Autodesk Inventor part; units mm, degrees
ref_plane "YZ Plane" through (0, 0, 0) normal (1, 0, 0) x (0, 1, 0)
ref_plane "XZ Plane" through (0, 0, 0) normal (0, 1, 0) x (-1, 0, 0)
ref_plane "XY Plane" through (0, 0, 0) normal (0, 0, 1) x (1, 0, 0)
sketch "Sketch1" plane through (0, 0, 0) normal (0, 0, 1) x (1, 0, 0)
  line L0 (0, 0) -> (152.4, 0)
  line L1 (152.4, 0) -> (152.4, 3.175)
  line L2 (152.4, 3.175) -> (0, 3.175)
  line L3 (0, 3.175) -> (0, 0)
  line L4 (0, 3.175) -> (11.1125, 3.175)
  line L5 (152.4, 3.175) -> (190.5, 3.175)
  line L6 (0, 3.175) -> (11.1125, 3.175)
  line L7 (0, 3.175) -> (-3.175, 3.175)
  line L8 (-3.175, 3.175) -> (-3.175, 485.775)
  line L9 (-3.175, 485.775) -> (0, 485.775)
  line L10 (0, 485.775) -> (0, 3.175)
  line L11 (-3.175, 40.7756) -> (-6.35, 40.7756)
  line L12 (-6.35, 40.7756) -> (-6.35, 421.7756)
  line L13 (-6.35, 421.7756) -> (-3.175, 421.7756)
  line L14 (-3.175, 421.7756) -> (-3.175, 40.7756)
  line L15 (190.5, 3.175) -> (-3.175, 485.775)
  line L16 (165.1, 3.175) -> (165.1, 66.675)
  line L17 (165.1, 3.175) -> (228.6, 3.175) construction
  point P0 (5.5563, 3.175)
  point P1 (-1.5875, 3.175)
  point P2 (-4.7625, 40.7756)
  point P3 (-3.175, 421.7756)
  point P4 (165.1, 66.4668)
  dimension "d0" = 152.4
  dimension "d1" = 3.175
  dimension "d7" = 38.1
  dimension "d15" = 3.175
  dimension "d16" = 482.6
  dimension "d17" = 3.175
  dimension "d18" = 381
  dimension "d19" = 37.6006
  dimension "d20" = 63.5
  dimension "d21" = 90
  dimension "d22" = 25.4
extrude "Extrusion1" add sketch "Sketch1" along normal blind 3.175 contours L3 L2 L1 L0 | L10 L15 L16 L5 L2 | L7 L8 L15 L10 | L11 L12 L13 L8
properties part number "side support"
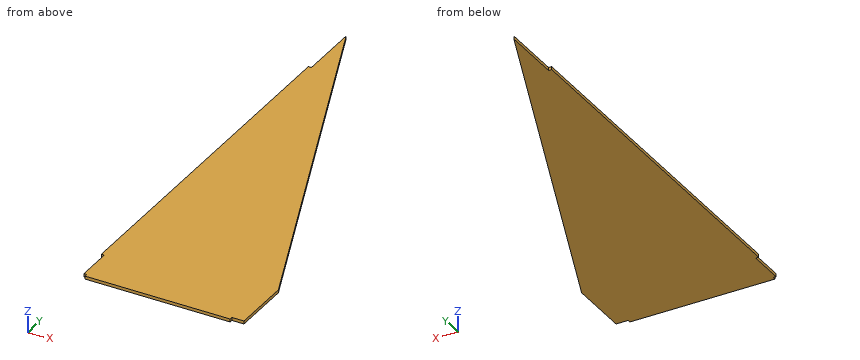
Work out the finished part from the listing and answer in its coordinate system (mm). Give positions to 0.01 mm unless a question says otherwise; leave off trailing zeros. Write each loop counter-clockwise with the first axis right and the second up, starting at its lowest first coordinate (ties: lowest second). Pieces come first, ordered by that corner, then holes. Notation, with made-up numbers: (75, -39.5) -> (97, -39.5) arc R21 cw to (97, -0.5) -> close; hole circle Ø4 at (82, 4.5). An arc over 180 degrees is marked (long way). Write item = value, one per line.
Q1. Section C-C on x = 116 is taken. Determine the outline of the cut face in (y, z) (3 decimals).
Computed values:
outline = (0, 0) -> (188.814, 0) -> (188.814, 3.175) -> (0, 3.175) -> close
Q2. Section A-A on z = 0.9 is taken. Determine the outline of the cut face in (x, y) (3 decimals).
Computed values:
outline = (-6.35, 40.776) -> (-3.175, 40.776) -> (-3.175, 3.175) -> (0, 3.175) -> (0, 0) -> (152.4, 0) -> (152.4, 3.175) -> (165.1, 3.175) -> (165.1, 66.467) -> (-3.175, 485.775) -> (-3.175, 421.776) -> (-6.35, 421.776) -> close
Q3. Flat-ended cylindrical pins translate along their axes: pin 1 Ø1 at (x, z) = (53.5, 1.5) entering from +Y; pin 2 Ø1 at (x, z) = (-4.5, 1) entering from -Y; pin 3 Ø1.5 at (y, z) = (85.5, 2) entering from +X. Find the tip coordinate at first contact, or state that the pin passes through.
Computed values:
pin_1 = 345.8
pin_2 = 40.78
pin_3 = 157.76
Q4. Consider line 1 along Y through (x, z) = (19, 1.1); line 2 along Y through (x, z) = (51, 2.4); line 3 along X through (y, z) = (377.5, 2.7). Determine where each line is inside the solid, lowest interval first.
Computed values:
line_1 = 0 to 430.52
line_2 = 0 to 350.78
line_3 = -6.35 to 40.28
Q5. Section B-B on y = 445 is taken. Determine the outline of the cut face in (x, z) (3 decimals).
Computed values:
outline = (-3.175, 0) -> (13.189, 0) -> (13.189, 3.175) -> (-3.175, 3.175) -> close
